Read the model definition and answer for the solid it produces. Units are mm, in the model's axes. Give positions to 0.01 mm unless a question says otherwise; leave off trailing zeros. Loops run counter-clockwise (first coordinate to the right, second up) from the corner with the lowest first, then second, coordinate; pieces in that order, holes last. Notation, with made-up numbers: (13, 5) - (22, 5) arc R23 cw to (22, 41) - close; hole circle Ø7 at (6.5, 85.5). An arc over 180 degrees is marked (long way). Put each result on its own line as item: value. Start each with the question number.
1. A cutting plane is placed at D-D, the plane x = 23. Determine the outline of the cut face in (y, z), plus the area to 3 significant figures.
2. A cutting plane is placed at C-C, the plane z = -29.5. Determine the outline of the cut face in (x, y).
3. A cutting plane is placed at B-B, the plane x = -14.5. Determine the outline of the cut face in (y, z), plus the area to 3 significant figures.
4. Given pin 1 Ø12 at (x, z) = (15, -60) entering from +Y; pin 2 Ø1.5 at (x, y) = (-13.5, 3) entering from -Z; pin 3 Ø0.8 at (x, y) = (-14.5, 0.5) entering from +Z, each flat-ended and moving along its own axis, determine where each tip first touches the part or whether it passes through.
5. A cutting plane is placed at A-A, the plane y = 2.65. Determine the outline of the cut face in (x, z), plus the area to 3 significant figures.
6. Consider L1, parallel to X at y = 3.9, z = 4; L2, parallel to Y at x = -6.5, z = -61; L3, parallel to Z at x = 5, y = 4.65. Determine where each line is inside the solid, lowest interval first. Write a range as from..to.
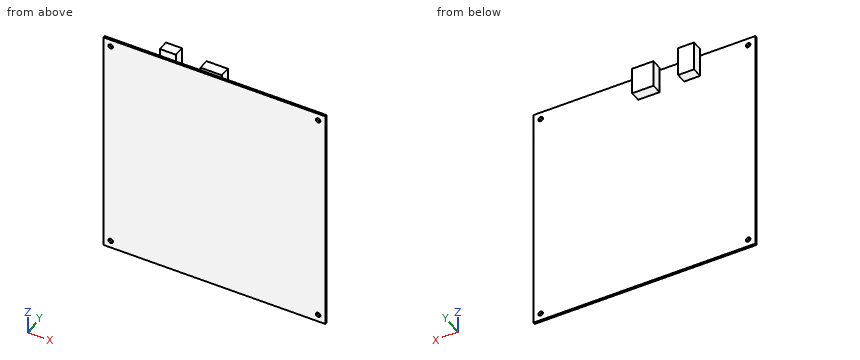
```python
from build123d import *

# Parameters (mm, degrees)
SKETCH1_W           = 106
SKETCH1_H           = 110
SKETCH1_R           = 1.1
BOSS_EXTRUDE1_DEPTH = 1
BOSS_EXTRUDE3_DEPTH = 5
SKETCH3_W           = 10.16
SKETCH3_H           = 13
BOSS_EXTRUDE4_DEPTH = 5


with BuildPart() as part:
    # Sketch1 → Boss-Extrude1 (new body)
    with BuildSketch(Plane(origin=(0, 0, 0), x_dir=(1, 0, 0), z_dir=(0, 1, 0))):
        with Locations((8.955727632, 44.943820005)):
            Rectangle(SKETCH1_W, SKETCH1_H)
        with Locations(Location((-40.544272368, -6.556179995, 0), (0, 0, 270))):
            Circle(SKETCH1_R, mode=Mode.SUBTRACT)
        with Locations(Location((58.455727632, -6.556179995, 0), (0, 0, 270))):
            Circle(SKETCH1_R, mode=Mode.SUBTRACT)
        with Locations(Location((-40.544272368, 96.443820005, 0), (0, 0, 270))):
            Circle(SKETCH1_R, mode=Mode.SUBTRACT)
        with Locations(Location((58.455727632, 96.443820005, 0), (0, 0, 270))):
            Circle(SKETCH1_R, mode=Mode.SUBTRACT)
    extrude(amount=BOSS_EXTRUDE1_DEPTH)

    # 3DSketch1 → Boss-Extrude3 (add)
    with BuildSketch(Plane(origin=(-17.624272368, 1, -0.613820005), x_dir=(0.47206668121683765, 0, 0.8815628443196325), z_dir=(0, -1, 0))):
        Polygon((0, 0), (3.597148111, -6.717508874), (16.141787386, 0), (12.544639275, 6.717508874), align=None)
    extrude(amount=-BOSS_EXTRUDE3_DEPTH)

    # Sketch3 → Boss-Extrude4 (add)
    with BuildSketch(Plane(origin=(0, 1, 0), x_dir=(1, 0, 0), z_dir=(0, 1, 0))):
        with Locations((6.825727632, -4.886179995)):
            Rectangle(SKETCH3_W, SKETCH3_H)
    extrude(amount=BOSS_EXTRUDE4_DEPTH)


solid = part.part
```
Return value:
1. outline: (0, -99.94) - (1, -99.94) - (1, 10.06) - (0, 10.06) - close
1. area: 110 mm2
2. outline: (-44.04, 0) - (61.96, 0) - (61.96, 1) - (-44.04, 1) - close
3. outline: (0, -99.94) - (1, -99.94) - (1, -0.61) - (6, -0.61) - (6, 13.62) - (1, 13.62) - (1, 10.06) - (0, 10.06) - close
3. area: 181 mm2
4. pin 1: stops at y = 1
4. pin 2: stops at z = -0.61
4. pin 3: stops at z = 10.06
5. outline: (-17.62, -0.61) - (-10, -0.61) - (-10, 13.62) - (-17.62, 13.62) - close; (1.75, -1.61) - (11.91, -1.61) - (11.91, 11.39) - (1.75, 11.39) - close
5. area: 241 mm2
6. L1: x = -17.62..-10, 1.75..11.91
6. L2: y = 0..1
6. L3: z = -1.61..11.39
